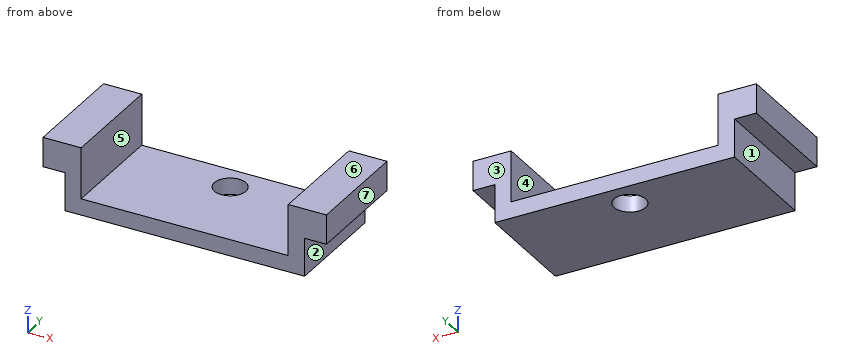
```python
from build123d import *

# Parameters (mm, degrees)
SKETCH1_W           = 19
SKETCH1_H           = 1.5
SKETCH1_W_2         = 1.5
SKETCH1_H_2         = 4
BOSS_EXTRUDE1_DEPTH = 5
SKETCH2_W           = 3.5
SKETCH2_H           = 2
BOSS_EXTRUDE2_DEPTH = 5
SKETCH3_R           = 1.45
CUT_EXTRUDE1_DEPTH  = 5
BOSS_EXTRUDE3_DEPTH = 5
SKETCH5_W           = 3.5
SKETCH5_H           = 10
BOSS_EXTRUDE4_DEPTH = 0.7


with BuildPart() as part:
    # Sketch1 → Boss-Extrude1 (new body)
    with BuildSketch(Plane(origin=(0, 0, 0), x_dir=(1, 0, 0), z_dir=(0, 1, 0))):
        with Locations((6.456445993, -4.406794425)):
            Rectangle(SKETCH1_W, SKETCH1_H)
        with Locations((-3.793554007, -4.406794425)):
            Rectangle(SKETCH1_W_2, SKETCH1_H)
        with Locations((-3.793554007, -7.156794425)):
            Rectangle(SKETCH1_W_2, SKETCH1_H_2)
        with Locations((16.706445993, -4.406794425)):
            Rectangle(SKETCH1_W_2, SKETCH1_H)
        with Locations((16.706445993, -7.156794425)):
            Rectangle(SKETCH1_W_2, SKETCH1_H_2)
    extrude(amount=BOSS_EXTRUDE1_DEPTH)

    # Sketch2 → Boss-Extrude2 (add)
    with BuildSketch(Plane(origin=(0, 5, 0), x_dir=(1, 0, 0), z_dir=(0, 1, 0))):
        with Locations((-4.793554007, -8.156794425)):
            Rectangle(SKETCH2_W, SKETCH2_H)
        with Locations((17.706445993, -8.156794425)):
            Rectangle(SKETCH2_W, SKETCH2_H)
    extrude(amount=-BOSS_EXTRUDE2_DEPTH)

    # Sketch3 → Cut-Extrude1 (cut)
    with BuildSketch(Plane.XY.offset(5.156794425)):
        with Locations((6.456445993, 2.5)):
            Circle(SKETCH3_R)
    extrude(amount=-CUT_EXTRUDE1_DEPTH, mode=Mode.SUBTRACT)

    # Sketch4 → Boss-Extrude3 (add)
    with BuildSketch(Plane.XZ):
        Polygon((17.456445993, 3.656794425), (17.456445993, 7.156794425), (19.456445993, 7.156794425), (19.456445993, 9.156794425), (15.956445993, 9.156794425), (15.956445993, 5.156794425), (-3.043554007, 5.156794425), (-3.043554007, 9.156794425), (-6.543554007, 9.156794425), (-6.543554007, 7.156794425), (-4.543554007, 7.156794425), (-4.543554007, 3.656794425), align=None)
    extrude(amount=BOSS_EXTRUDE3_DEPTH)

    # Sketch5 → Boss-Extrude4 (add)
    with BuildSketch(Plane.XY.offset(9.156794425)):
        with Locations((17.706445993, 0)):
            Rectangle(SKETCH5_W, SKETCH5_H)
        with Locations((-4.793554007, 0)):
            Rectangle(SKETCH5_W, SKETCH5_H)
    extrude(amount=BOSS_EXTRUDE4_DEPTH)


solid = part.part
```
Check sheet for the modelled part. Datum: model origin and axes. Units: mm. Face numbers are marked on the shaded views. A direction names the side the tool comes from. Coordinates: 2 decimals unless noted, no trailing zeros. Write each loop counter-clockwise with the first axis right and the second up, starting at its lowest first coordinate (ties: lowest second). Pieces come first, ordered by that corner, then holes. Notation, with made-up numbers: (-6, 79) - (15, 79) arc R21 ccw to (15, 93) - close; hole circle Ø7 at (-14.5, 70). An arc over 180 degrees is marked (long way). One line per question, with ' | ' between items.
Item 1: Sectioned sample at D-D on y = 2.75. Record the boundary of the cut face in (x, z).
Determined:
outline: (-6.54, 7.16) - (-4.54, 7.16) - (-4.54, 3.66) - (5.03, 3.66) - (5.03, 5.16) - (-3.04, 5.16) - (-3.04, 9.86) - (-6.54, 9.86) - close; (7.88, 3.66) - (17.46, 3.66) - (17.46, 7.16) - (19.46, 7.16) - (19.46, 9.86) - (15.96, 9.86) - (15.96, 5.16) - (7.88, 5.16) - close
Item 2: Sectioned sample at B-B on z = 4. Record the boundary of the cut face in (x, y), plus the area to 3 significant figures.
Determined:
outline: (-4.54, -5) - (17.46, -5) - (17.46, 5) - (-4.54, 5) - close; hole circle Ø2.9 at (6.46, 2.5) | area: 213 mm2
Item 3: Sectioned sample at C-C on y = -1. Record the boundary of the cut face in (x, z).
Determined:
outline: (-6.54, 7.16) - (-4.54, 7.16) - (-4.54, 3.66) - (17.46, 3.66) - (17.46, 7.16) - (19.46, 7.16) - (19.46, 9.86) - (15.96, 9.86) - (15.96, 5.16) - (-3.04, 5.16) - (-3.04, 9.86) - (-6.54, 9.86) - close
Item 4: Gauge pin test, flat ends, axial feed: P1, Ø6, axis at x = 3.5, y = 1, coming from the +Z side; P2, Ø1, axis at x = -5.5, y = 1, coming from the -Z side; P3, Ø1, axis at y = -1.5, z = 4.5, coming from the -X side; P4, Ø1.5, axis at x = -3, y = -1, coming from the +Z side. Record the tip position at first contact, or that the pin passes through.
Determined:
P1: stops at z = 5.16 | P2: stops at z = 7.16 | P3: stops at x = -4.54 | P4: stops at z = 9.86
Item 5: Thickness scan on line 1 (X direction, y = 2.75, z = 6); line 2 (X direction, y = -1.75, z = 8); line 3 (Z direction, x = 14.25, y = -0.75). Record the ranges inside material, lowest first. Write a range as [from, to].
Determined:
line 1: x = [-4.54, -3.04], [15.96, 17.46] | line 2: x = [-6.54, -3.04], [15.96, 19.46] | line 3: z = [3.66, 5.16]
Item 6: Sectioned sample at A-A on z = 7.5. Record the boundary of the cut face in (x, y), plus the area to 3 significant figures.
Determined:
outline: (-6.54, -5) - (-3.04, -5) - (-3.04, 5) - (-6.54, 5) - close; (15.96, -5) - (19.46, -5) - (19.46, 5) - (15.96, 5) - close | area: 70.0 mm2
Item 7: Mould release check, pull along X, two halves, no side actions. Record for the marked faces 5, 6 and 7: pulls with the +X half, pulls with the -X half, needs draft (parallel to the pull), parting line crosses it, or undercut.
Determined:
face 5: undercut | face 6: needs draft | face 7: pulls with the +X half
Item 8: Access from +Z, -Z, +X, -X, +Y, -Y to the whole of each face (thin tool, end or side, straight path). Record for the marked faces 1, 2, 3 and 4.
Determined:
face 1: -Z, -X, +Y, -Y | face 2: -Z, +X, +Y, -Y | face 3: +Z, -Z, +X, -X, +Y | face 4: +Z, +Y, -Y
